from build123d import *

# Parameters (mm, degrees)
F0_R     = 25
F0_R_2   = 21.2
F1_DEPTH = 5


with BuildPart() as f1:
    # F0 (on Front) → F1 (new body)
    with BuildSketch(Plane.XZ):
        Circle(F0_R)
        Circle(F0_R_2, mode=Mode.SUBTRACT)
    extrude(amount=F1_DEPTH)

    # F2 (on Top) → F3 (revolve)
    with BuildSketch(Plane.XY):
        with BuildLine():
            Line((17.6, 4.5), (17.6, 0.5))
            ThreePointArc((17.6, 0.5), (17.746447, 0.146447), (18.1, 0))
            Line((18.1, 0), (25, 0))
            Line((25, 0), (25, 1))
            ThreePointArc((25, 1), (23.828427, 3.828427), (21, 5))
            Line((21, 5), (18.1, 5))
            ThreePointArc((18.1, 5), (17.746447, 4.853553), (17.6, 4.5))
        make_face()
    revolve(axis=Axis((0, 0, 0), (0, -1, 0)))


solid = f1.part
Input: part model. Units: mm. Frame: model coordinates. A direction names the side the tool comes from. Give positions to 0.01 mm unless a question says otherwise; leave off trailing zeros. Order: outer loops, then holes, each group sorted by start corner. A loop starts at its lowest first (then second) coordinate and runs counter-clockwise, first axis right, second up.
Q1. Section A-A on x = 0. Output: boundary loops of the cut face in (y, z).
Checked values:
outline: (-5, -25) - (1, -25) arc R4 ccw to (5, -21) - (5, -18.1) arc R0.5 ccw to (4.5, -17.6) - (0.5, -17.6) arc R0.5 ccw to (0, -18.1) - (0, -21.2) - (-5, -21.2) - close; (-5, 21.2) - (0, 21.2) - (0, 18.1) arc R0.5 ccw to (0.5, 17.6) - (4.5, 17.6) arc R0.5 ccw to (5, 18.1) - (5, 21) arc R4 ccw to (1, 25) - (-5, 25) - close
Q2. Set-up query: faces 4 (the flat face through (-11.2, -5, -18.4)), 5 (the cylindrical face through (19.583, -2.465, -8.12)). Return all of +Z, -Z, +X, -X, +Y, -Y with unobstructed straight access to the full face (end or side cutting, diameter ignored); none if empty.
Checked values:
face 4: +Z, -Z, +X, -X, -Y
face 5: -Y
Q3. Ray query, probe 1 along X at (y, z) = (0.5, -0.5) (3 decimals); probe 2 along Z at (x, y) = (0, -2.1); probe 3 along Y at (x, z) = (-19, -6.5). Return the intervals inside material, ascending.
Checked values:
probe 1: x = -24.995 to -17.593, 17.593 to 24.995
probe 2: z = -25 to -21.2, 21.2 to 25
probe 3: y = 0 to 5
Q4. Draft query along Z for faces 1 (the cylindrical face through (16.787, 2.472, 5.287)), 2 (the cylindrical face through (23.846, -1.958, 7.509)), 3 (the flat face through (9, 5, 16)). Return one class per face: +Z half, -Z half, draft (parallel to the pull), parting line (faces both ways), or undercut.
Checked values:
face 1: undercut
face 2: parting line
face 3: draft
Q5. Section B-B on y = 1.75. Output: boundary loops of the cut face in (x, z), and give its area (3 significant figures).
Checked values:
outline: circle Ø49.86 at (0, 0); hole circle Ø35.2 at (0, 0)
area: 979 mm2
Q6. Contact query for flat-ended pins moving along their axis: pin 1 Ø1.5 at (x, y) = (5.5, 0) entering from +Z; pin 2 Ø6 at (y, z) = (-3.5, -9.5) entering from +X; pin 3 Ø1.5 at (y, z) = (1, 10.5) entering from -X. Output: stop coordinate, or through.
Checked values:
pin 1: stops at z = 24.54
pin 2: stops at x = 24.14
pin 3: stops at x = -23.02
